Autodesk Inventor part; units mm, degrees
ref_plane "YZ Plane" through (0, 0, 0) normal (1, 0, 0) x (0, 1, 0)
ref_plane "XZ Plane" through (0, 0, 0) normal (0, 1, 0) x (-1, 0, 0)
ref_plane "XY Plane" through (0, 0, 0) normal (0, 0, 1) x (1, 0, 0)
sketch "Boceto1" plane through (0, 0, 0) normal (0, 1, 0) x (-1, 0, 0)
  circle A0 centre (0, 0) radius 10
  dimension "d0" = 20
extrude "Extrusión1" add sketch "Boceto1" along normal blind 2
sketch "Boceto2" plane through (0, 2, 0) normal (0, 1, 0) x (1, 0, 0)
  line L0 (-3, -6) -> (3, -6)
  line L1 (6, -3) -> (6, 3)
  line L2 (3, 6) -> (-3, 6)
  line L3 (-6, 3) -> (-6, -3)
  arc A0 (-3, 6) -> (-6, 3) centre (-3, 3) ccw
  arc A1 (-6, -3) -> (-3, -6) centre (-3, -3) ccw
  arc A2 (3, -6) -> (6, -3) centre (3, -3) ccw
  arc A3 (6, 3) -> (3, 6) centre (3, 3) ccw
  point P0 (0, 0)
  point P1 (-6, -6)
  point P2 (6, 6)
  point P3 (-6, 6)
  point P4 (0, 6)
  point P5 (-6, 0)
  dimension "d3" = 12
  dimension "d4" = 12
  dimension "d5" = 3
extrude "Extrusión2" add sketch "Boceto2" along normal blind 10
sketch "Boceto3" plane through (0, 12, 0) normal (0, 1, 0) x (1, 0, 0)
  circle A0 centre (0, 0) radius 5
  dimension "d8" = 10
extrude "Extrusión3" add sketch "Boceto3" along normal blind 2
sketch "Boceto4" plane through (0, 0, 0) normal (0, -1, 0) x (1, 0, 0)
  circle A0 centre (0, 0) radius 3
  dimension "d11" = 6
extrude "Extrusión4" cut sketch "Boceto4" against normal blind 12
chamfer "Chaflán1" distance 0.2 angle 45 11 edges at (-5, 14, 0) (6, 12, 0) (5.1213, 12, -5.1213) (0, 12, -6) (-5.1213, 12, -5.1213) (-6, 12, 0) (-5.1213, 12, 5.1213) (0, 12, 6) (5.1213, 12, 5.1213) (10, 2, 0) (10, 0, 0)
properties part number "Front_bush"
The listing builds one solid part. Answer for the finished solid, in the listing's coordinates (mm). A direction names the side the tool comes from. Round coordinates to 2 decimals unless told otherwise and drop trailing zeros. Write each loop counter-clockwise with the first axis right and the second up, starting at its lowest first coordinate (ties: lowest second). Pieces come first, ordered by that corner, then holes. Notation, with made-up numbers: (-37.75, 52) - (-23.75, 52) arc R21 cw to (-23.75, 66) - close; hole circle Ø2 at (75, 44.5). An arc over 180 degrees is marked (long way). Use a Markdown table: item, result. Add a question column.
1. A tool of negligible diameter and unlimited length cuts with its end or side. For faces 5 (the face through (-5.1, 6.83, 5.14)), 6 (the face through (5.1, 6.83, -5.14)), 7 (the face through (0.1, 2, -6.4)), 8 (the face through (0, 7, -6)), from which of +Z, -Z, +X, -X, +Y, -Y can it reach the whole face along a straight path? Write none if from no direction.
2. For a pull along X with two mould halves and no side action, classify faces 1 (the face through (-3, 6, 0)), 2 (the face through (5.14, 6.83, 5.1)), 3 (the face through (-1.08, 12.89, -4.88)), 4 (the face through (0, 7, 6)) as +X half, -X half, draft (parallel to the pull), parting line (faces both ways), or undercut.
3. Flat-ended cylindrical pins translate along their axes: P1, Ø5.5, axis at x = 0, z = 0, coming from the -Y side; P2, Ø2, axis at y = 9.5, z = -1.5, coming from the -X side; P3, Ø3, axis at x = 1.5, y = 7, coming from the -Z side. Find the tip coordinate at first contact, or state that the pin passes through.
4. The part is cut by section A-A (x = 0). Write down the section's boundary in (y, z).
5. The part is cut by section C-C (z = 0). Write down the section's boundary in (x, y).
6. Consider line 1 (Z direction, x = 0, y = 5.5); line 2 (X direction, y = 6.25, z = -0.5); line 3 (Y direction, x = 7.75, z = 4). Determine where each line is inside the solid, lowest interval first.
7. The part is cut by section B-B (y = 9.25). Write down the section's boundary in (x, z), and give its area (3 significant figures).
8. The part is cut by section D-D (y = 13). Write down the section's boundary in (x, z), and give its area (3 significant figures).
Reported:
| question | item | result |
|---|---|---|
| 1 | face 5 | +Z, -X, +Y |
| 1 | face 6 | -Z, +X, +Y |
| 1 | face 7 | +Y |
| 1 | face 8 | -Z, +X, -X, +Y |
| 2 | face 1 | undercut |
| 2 | face 2 | +X half |
| 2 | face 3 | parting line |
| 2 | face 4 | draft |
| 3 | P1 | y = 12 |
| 3 | P2 | x = -6 |
| 3 | P3 | z = -6 |
| 4 | outline | (0, -9.8) - (0.2, -10) - (1.8, -10) - (2, -9.8) - (2, -6) - (11.8, -6) - (12, -5.8) - (12, -5) - (13.8, -5) - (14, -4.8) - (14, 4.8) - (13.8, 5) - (12, 5) - (12, 5.8) - (11.8, 6) - (2, 6) - (2, 9.8) - (1.8, 10) - (0.2, 10) - (0, 9.8) - (0, 3) - (12, 3) - (12, -3) - (0, -3) - close |
| 5 | outline | (-10, 0.2) - (-9.8, 0) - (-3, 0) - (-3, 12) - (3, 12) - (3, 0) - (9.8, 0) - (10, 0.2) - (10, 1.8) - (9.8, 2) - (6, 2) - (6, 11.8) - (5.8, 12) - (5, 12) - (5, 13.8) - (4.8, 14) - (-4.8, 14) - (-5, 13.8) - (-5, 12) - (-5.8, 12) - (-6, 11.8) - (-6, 2) - (-9.8, 2) - (-10, 1.8) - close |
| 6 | line 1 | -6 to -3, 3 to 6 |
| 6 | line 2 | -6 to -2.96, 2.96 to 6 |
| 6 | line 3 | 0 to 2 |
| 7 | outline | (-6, -3) arc R3 ccw to (-3, -6) - (3, -6) arc R3 ccw to (6, -3) - (6, 3) arc R3 ccw to (3, 6) - (-3, 6) arc R3 ccw to (-6, 3) - close; hole circle Ø6 at (0, 0) |
| 7 | area | 108 mm^2 |
| 8 | outline | circle Ø10 at (0, 0) |
| 8 | area | 78.5 mm^2 |
